Print and shaded views of the part. All mm, measured from the part's lowest x, y and z. A direction names the side the tool comes from. Coordinates: 2 decimals unless noted, no trailing zeros. Order: outer loops, then holes, each group sorted by start corner. A loop starts at its lowest first (then second) coordinate and runs counter-clockwise, first axis right, second up.
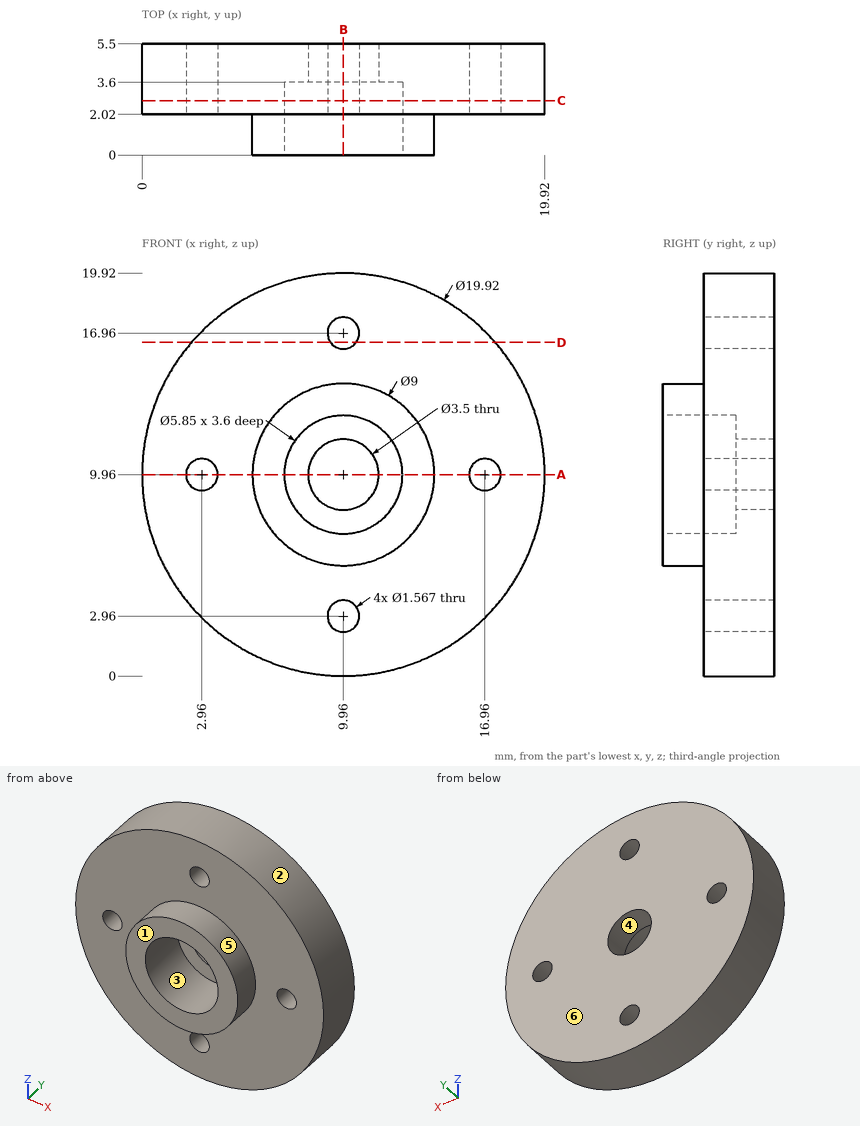
Q1. Cut at B-B, the plane x = 9.96. List the corners of the cut face in (y, z) (1 decimal), plus the area to 3 significant figures.
Established:
outline: (0, 5.5) - (2, 5.5) - (2, 3.7) - (5.5, 3.7) - (5.5, 8.2) - (3.6, 8.2) - (3.6, 7) - (0, 7) - close; (0, 12.9) - (3.6, 12.9) - (3.6, 11.7) - (5.5, 11.7) - (5.5, 16.2) - (2, 16.2) - (2, 14.5) - (0, 14.5) - close; (2, 0) - (5.5, 0) - (5.5, 2.2) - (2, 2.2) - close; (2, 17.7) - (5.5, 17.7) - (5.5, 19.9) - (2, 19.9) - close
area: 48.9 mm2
Q2. Probe line 1 (Z direction, x = 9.96, y = 2.3) (1 decimal); line 2 (Z direction, x = 9.96, y = 3.8); line 3 (Y direction, x = 8.25, z = 3). List the from-to ranges inside material, lowest first.
Established:
line 1: z = 0 to 2.2, 3.7 to 7, 12.9 to 16.2, 17.7 to 19.9
line 2: z = 0 to 2.18, 3.74 to 8.21, 11.71 to 16.18, 17.74 to 19.92
line 3: y = 2.02 to 5.5
Q3. Cut at A-A, the plane z = 9.96. List the corners of the cut face in (x, y) (1 decimal).
Established:
outline: (0, 2) - (2.2, 2) - (2.2, 5.5) - (0, 5.5) - close; (3.7, 2) - (5.5, 2) - (5.5, 0) - (7, 0) - (7, 3.6) - (8.2, 3.6) - (8.2, 5.5) - (3.7, 5.5) - close; (11.7, 3.6) - (12.9, 3.6) - (12.9, 0) - (14.5, 0) - (14.5, 2) - (16.2, 2) - (16.2, 5.5) - (11.7, 5.5) - close; (17.7, 2) - (19.9, 2) - (19.9, 5.5) - (17.7, 5.5) - close
Q4. Drop flat-ended pins along their axis: P1, Ø4.5, axis at x = 9.96, z = 9.96, coming from the -Y side; P2, Ø9.5, axis at x = 9.96, z = 9.96, coming from the +Y side; P3, Ø1, axis at x = 17.5, y = 5, coming from the -Z side; P4, Ø2, axis at y = 2.5, z = 5, coming from the +X side. Give the stop position or say it passes through.
Established:
P1: stops at y = 3.6
P2: stops at y = 5.5
P3: stops at z = 2.91
P4: stops at x = 19.1
Q5. Which spindle directions (+Z, -Z, +X, -X, +Y, -Y) get a long thin tool onto all of the face, cutting with end or side? Do the marked faces 5 and 6. Say none if no direction does.
Established:
face 5: -Y
face 6: +Z, -Z, +X, -X, +Y
Q6. Cut at D-D, the plane z = 16.5. List the corners of the cut face in (x, y), plus the area to 3 significant figures.
Established:
outline: (2.45, 2.02) - (9.33, 2.02) - (9.33, 5.5) - (2.45, 5.5) - close; (10.59, 2.02) - (17.47, 2.02) - (17.47, 5.5) - (10.59, 5.5) - close
area: 47.9 mm2
Q7. Mould opens along Z. For the marked faces 1, 2, 3 and 4 say: pulls with the +Z half, pulls with the -Z half, needs draft (parallel to the pull), parting line crosses it, or undercut.
Established:
face 1: needs draft
face 2: parting line crosses it
face 3: undercut
face 4: undercut
Q8. Cut at C-C, the plane y = 2.7. Count the separate pieces of the cut face and the enclosed holes in it, plus the area to 3 significant figures.
Established:
separate pieces: 1
enclosed holes: 5
area: 277 mm2
